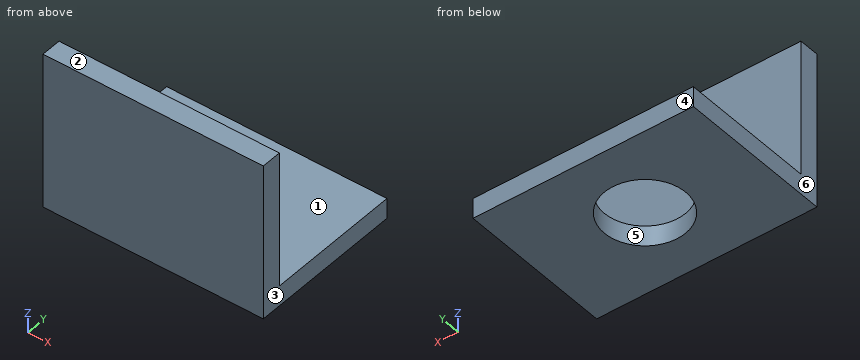
```python
from build123d import *

# Parameters (mm, degrees)
ESQUISSE1_W        = 38
ESQUISSE1_H        = 23.5
ESQUISSE1_R        = 7
BOSS_EXTRU_1_DEPTH = 3.5
ESQUISSE1_4_W      = 38
ESQUISSE1_4_H      = 3.5
BOSS_EXTRU_2_DEPTH = 27


with BuildPart() as part:
    # Esquisse1 → Boss.-Extru.1 (new body)
    with BuildSketch(Plane.XY):
        with Locations((0, 15.25)):
            Rectangle(ESQUISSE1_W, ESQUISSE1_H)
        with Locations((0, 13.5)):
            Circle(ESQUISSE1_R, mode=Mode.SUBTRACT)
    extrude(amount=BOSS_EXTRU_1_DEPTH)

    # Esquisse1<4> → Boss.-Extru.2 (add)
    with BuildSketch(Plane.XY):
        with Locations((0, 1.75)):
            Rectangle(ESQUISSE1_4_W, ESQUISSE1_4_H)
    extrude(amount=BOSS_EXTRU_2_DEPTH)


solid = part.part
```
Can you work these out from the model? Positions are in its coordinate system, mm. Face numbers are marked on the shaded views. A direction names the side the tool comes from. Coordinates: 2 decimals unless noted, no trailing zeros. Loops run counter-clockwise (first coordinate to the right, second up) from the corner with the lowest first, then second, coordinate; pieces in that order, holes last.
Item 1: Suppose I cut it at D-D (z = 23.75). Please give me the cut outline in (x, y).
Answers below:
outline: (-19, 0) - (19, 0) - (19, 3.5) - (-19, 3.5) - close
Item 2: Suppose I cut it at A-A (x = 0). Please give me the cut outline in (y, z), then the cut area to 3 significant figures.
Answers below:
outline: (0, 0) - (6.5, 0) - (6.5, 3.5) - (3.5, 3.5) - (3.5, 27) - (0, 27) - close; (20.5, 0) - (27, 0) - (27, 3.5) - (20.5, 3.5) - close
area: 128 mm2
Item 3: I'm going to push a flat-ended pin straight in: pin 1 (12 mm diameter, centred on x = 7, z = 11, fed in from +Y). Where does the tip first touch, or does it pass through?
Answers below:
pin 1: stops at y = 3.5
Item 4: Suppose I cut it at B-B (y = 13.5). Please give me the cut outline in (x, z), then the cut area to 3 significant figures.
Answers below:
outline: (-19, 0) - (-7, 0) - (-7, 3.5) - (-19, 3.5) - close; (7, 0) - (19, 0) - (19, 3.5) - (7, 3.5) - close
area: 84.0 mm2
Item 5: Suppose I cut it at C-C (x = 7.5). Please give me the cut outline in (y, z).
Answers below:
outline: (0, 0) - (27, 0) - (27, 3.5) - (3.5, 3.5) - (3.5, 27) - (0, 27) - close
Item 6: Which directions (+Z, -Z, +X, -X, +Y, -Y) give clear straight access to the entire face, cutting with the end or side of a thin tool? Please do the marked faces 1 and 2.
Answers below:
face 1: +Z, +X, -X, +Y
face 2: +Z, +X, -X, +Y, -Y
Item 7: If we mould it in two halves opening along X, with no side actions, what happens to the marked faces 3, 4, 5 and 6? For each: released by +X, released by -X, zero draft, split by the parting line, or undercut.
Answers below:
face 3: released by +X
face 4: zero draft
face 5: undercut
face 6: released by -X
Item 8: Please list where these lines run through material, in increasing order: L1, parallel to Y at x = 0, z = 1.1; L2, parallel to Z at x = -14, y = 22.5.
Answers below:
L1: y = 0 to 6.5, 20.5 to 27
L2: z = 0 to 3.5
